```python
from build123d import *

# Parameters (mm, degrees)
SKETCH_1_W                = 60
SKETCH_1_H                = 60
EXTRUDE_1_DEPTH           = 19.6
CHAMFER_1_SIZE            = 2
SKETCH_2_W                = 35
SKETCH_2_H                = 35
EXTRUDE_2_DEPTH           = 0.4
FILLET_1_R                = 2
HOLE_WIZARD_1_D           = 3.4
HOLE_WIZARD_1_CBORE_D     = 6
HOLE_WIZARD_1_CBORE_DEPTH = 5
HOLE_WIZARD_M3_1_D        = 2.5
HOLE_WIZARD_M3_1_DEPTH    = 3.5
HOLE_WIZARD_M3_1_TIP      = 0.751075774


with BuildPart() as part:
    # 草图1 → 凸台-拉伸1 (new body)
    with BuildSketch(Plane.XY):
        Rectangle(SKETCH_1_W, SKETCH_1_H)
    extrude(amount=EXTRUDE_1_DEPTH)

    # 倒角1
    chamfer_1_edges = [part.edges().sort_by_distance(p)[0] for p in [
        (30, -30, 9.8),
        (-30, -30, 9.8),
        (-30, 30, 9.8),
        (30, 30, 9.8),
    ]]
    chamfer(chamfer_1_edges, length=CHAMFER_1_SIZE)

    # 草图2 → 凸台-拉伸2 (add)
    with BuildSketch(Plane.XY.offset(19.6)):
        Rectangle(SKETCH_2_W, SKETCH_2_H)
    extrude(amount=EXTRUDE_2_DEPTH)

    # 圆角1
    fillet_1_edges = [part.edges().sort_by_distance(p)[0] for p in [
        (17.5, -17.5, 19.8),
        (17.5, 17.5, 19.8),
        (-17.5, 17.5, 19.8),
        (-17.5, -17.5, 19.8),
    ]]
    fillet(fillet_1_edges, radius=FILLET_1_R)

    # 孔1 (through all)
    with Locations(Plane(origin=(-25, 25, 19.6), x_dir=(1, 0, 0), z_dir=(0, 0, 1))):
        with Locations((0, 0), (50, 0), (0, -50), (50, -50)):
            CounterBoreHole(HOLE_WIZARD_1_D / 2, HOLE_WIZARD_1_CBORE_D / 2, HOLE_WIZARD_1_CBORE_DEPTH)

    # M3 螺纹孔1
    with Locations(Plane(origin=(-12.5, 12.5, 20), x_dir=(1, 0, 0), z_dir=(0, 0, 1))):
        with Locations((0, 0), (25, 0), (25, -25), (0, -25)):
            Hole(HOLE_WIZARD_M3_1_D / 2, depth=HOLE_WIZARD_M3_1_DEPTH)
            with Locations((0, 0, -(HOLE_WIZARD_M3_1_DEPTH + HOLE_WIZARD_M3_1_TIP / 2))):  # 118° drill point
                Cone(0, HOLE_WIZARD_M3_1_D / 2, HOLE_WIZARD_M3_1_TIP, mode=Mode.SUBTRACT)


solid = part.part
```
Model file for the job. Use its own axes, mm. A direction names the side the tool comes from. Coordinates: 2 decimals unless noted, no trailing zeros. Order: outer loops, then holes, each group sorted by start corner. A loop starts at its lowest first (then second) coordinate and runs counter-clockwise, first axis right, second up. Notation, with made-up numbers: M 15,37.25 L 36,37.25 A6 ccw 36,44.25 Z; hole C 9,-32 d2. An arc over 180 degrees is marked long. Answer as CSV lines item,"result".
(1) 3-axis set-ups, long thin cutter, end or side, ignore diameter. For faces 1 (the cylindrical face through (-25.914, -23.567, 7.198)), 2 (the flat face through (-25, 23, 14.6)), 3 (the cylindrical face through (-16.9, -16.93, 19.8)): which of +Z, -Z, +X, -X, +Y, -Y reach the whole face in a straight line?
Geometry says:
face 1,"+Z, -Z"
face 2,"+Z"
face 3,"+Z, -X, -Y"
(2) Band-saw the part on A-A, the plane x = -25. List the corners of the cut face in (y, z), then the cut area to 3 significant figures.
Geometry says:
outline,"M -30,0 L -26.7,0 L -26.7,14.6 L -28,14.6 L -28,19.6 L -30,19.6 Z; M -23.3,0 L 23.3,0 L 23.3,14.6 L 22,14.6 L 22,19.6 L -22,19.6 L -22,14.6 L -23.3,14.6 Z; M 26.7,0 L 30,0 L 30,19.6 L 28,19.6 L 28,14.6 L 26.7,14.6 Z"
area,"1,020 mm2"
(3) Band-saw the part on B-B, the plane z = 18. State how many separate pieces and enclosed holes the cut face has, then the cut area to 3 significant figures.
Geometry says:
separate pieces,"1"
enclosed holes,"8"
area,"3,460 mm2"
(4) Wall check: line 1 along Y through (x, z) = (12.5, 17.7); line 2 along Y through (x, z) = (25, 11.25); line 3 along Z through (x, y) = (-19.5, 18.5). Give the ranges that are in metal, low to high.
Geometry says:
line 1,"y = -30 to -13.75, -11.25 to 11.25, 13.75 to 30"
line 2,"y = -30 to -26.7, -23.3 to 23.3, 26.7 to 30"
line 3,"z = 0 to 19.6"
(5) Flat gauge pins, fed straight in: pin 1 (7 mm diameter, centred on x = -25, y = -25, fed in from +Z); pin 2 (2.5 mm diameter, centred on x = 25, y = -25, fed in from -Z) (3 decimals); pin 3 (1.8 mm diameter, centred on x = -25, y = -26.5, fed in from +Z). Where does each tip first touch, or does it go through?
Geometry says:
pin 1,"stops at z = 19.6"
pin 2,"passes through"
pin 3,"stops at z = 14.6"
(6) Pull direction X, two halves, no side cores. Call faces 4 (the flat face through (-25, -27, 14.6)), 5 (the flat face through (29, 29, 10)), 6 (the cylindrical face through (12.66, 13.74, 18.23)), 7 (the flat face through (0, 0, 20)): +X half, -X half, draft (parallel to the pull), parting line (faces both ways), or undercut.
Geometry says:
face 4,"undercut"
face 5,"+X half"
face 6,"undercut"
face 7,"draft"
